Part model, mm, in its own coordinate system. Face numbers are marked on the shaded views. A direction names the side the tool comes from. Round coordinates to 2 decimals unless told otherwise and drop trailing zeros. Loops run counter-clockwise (first coordinate to the right, second up) from the corner with the lowest first, then second, coordinate; pieces in that order, holes last. Notation, with made-up numbers: (45.25, -16) -> (99.25, -16) arc R19 cw to (99.25, 14) -> close; hole circle Ø9 at (56.5, 55). An arc over 180 degrees is marked (long way). Use a Markdown table: item, result. Add a question column.
Item 1: Which spindle directions (+Z, -Z, +X, -X, +Y, -Y) get a long thin tool onto all of the face, cutting with end or side? Do the marked faces 4, 5, 6, 7 and 8. Say none if no direction does.
Item 2: Cut at B-B, the plane y = 17. List the corners of the cut face in (x, z).
Item 3: Probe line 1 (Z direction, x = -94, y = 8); line 2 (X direction, y = 40, z = -35); line 3 (X direction, y = 12, z = -24). List the from-to ranges inside material, lowest first. Write a range as [from, to].
Item 4: Cut at D-D, the plane z = -29.5. List the corners of the cut face in (x, y), plus the area to 3 significant figures.
Item 5: Cut at A-A, the plane x = -80.5. List the corners of the cut face in (y, z).
Item 6: Flat gauge pin, fed straight in: pin 1 (1.5 mm diameter, centred on x = -68.5, z = -37.5, fed in from -Y). Where does the tip first touch, or does it go through?
Item 7: Two-plate mould, pull along X, no slides. Class the marked faces 1, 2 and 3: pulls with the +X half, pulls with the -X half, needs draft (parallel to the pull), parting line crosses it, or undercut.
Item 8: Cut at C-C, the plane z = -48.5. List the corners of the cut face in (x, y).
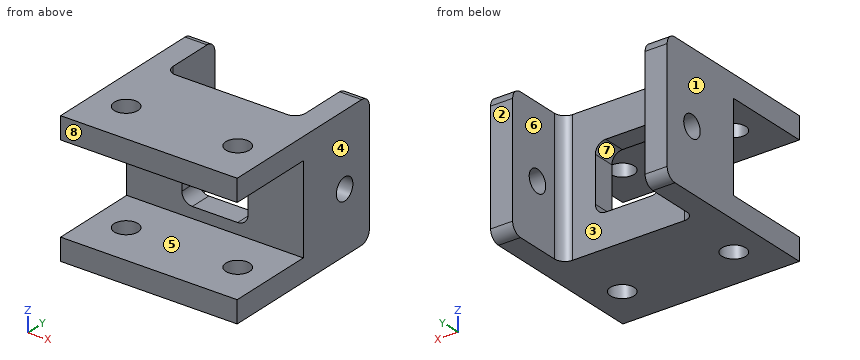
```python
from build123d import *

# Parameters (mm, degrees)
SKETCH1_W               = 50.8
SKETCH1_H               = 38.1
BOSS_EXTRUDE1_DEPTH     = 31.75
SKETCH2_W               = 25.4
SKETCH2_H               = 25.4
CUT_EXTRUDE1_DEPTH      = 85.79053849
SKETCH3_W               = 6.35
SKETCH3_H               = 38.1
BOSS_EXTRUDE2_DEPTH     = 19.05
SKETCH4_W               = 6.35
SKETCH4_H               = 38.1
BOSS_EXTRUDE3_DEPTH     = 19.05
CUT_EXTRUDE2_DEPTH      = 91.317082645
CUT_EXTRUDE2_DEPTH_BACK = 91.317082645
SKETCH5_R               = 3.175
FILLET1_R               = 3
SKETCH6_R               = 3.429
CUT_EXTRUDE3_DEPTH      = 127.788108172
SKETCH7_R               = 3.429
CUT_EXTRUDE4_DEPTH      = 127.788108172
SKETCH8_W               = 19.05
SKETCH8_H               = 19.05
CUT_EXTRUDE5_DEPTH      = 130.041736625
FILLET2_R               = 3
FILLET3_R               = 3


with BuildPart() as part:
    # Sketch1 → Boss-Extrude1 (new body)
    with BuildSketch(Plane(origin=(0, 0, 0), x_dir=(1, 0, 0), z_dir=(0, 1, 0))):
        with Locations((-84.340486484, 40.956107335)):
            Rectangle(SKETCH1_W, SKETCH1_H)
    extrude(amount=BOSS_EXTRUDE1_DEPTH)

    # Sketch2 → Cut-Extrude1 (cut, through all)
    with BuildSketch(Plane(origin=(-58.940486484, 0, 0), x_dir=(0, 0, -1), z_dir=(1, 0, 0))):
        with Locations((40.956107335, 12.7)):
            Rectangle(SKETCH2_W, SKETCH2_H)
    extrude(amount=-CUT_EXTRUDE1_DEPTH, mode=Mode.SUBTRACT)

    # Sketch3 → Boss-Extrude2 (add)
    with BuildSketch(Plane(origin=(0, 31.75, 0), x_dir=(1, 0, 0), z_dir=(0, 1, 0))):
        with Locations((-106.565486484, 40.956107335)):
            Rectangle(SKETCH3_W, SKETCH3_H)
    extrude(amount=BOSS_EXTRUDE2_DEPTH)

    # Sketch4 → Boss-Extrude3 (add)
    with BuildSketch(Plane(origin=(0, 31.75, 0), x_dir=(1, 0, 0), z_dir=(0, 1, 0))):
        with Locations((-62.115486484, 40.956107335)):
            Rectangle(SKETCH4_W, SKETCH4_H)
    extrude(amount=BOSS_EXTRUDE3_DEPTH)

    # Sketch5 → Cut-Extrude2 (cut, two sides: drawn at the far end of the back side and taken through both)
    with BuildSketch(Plane(origin=(-103.390486484, 0, 0), x_dir=(0, 0, -1), z_dir=(1, 0, 0)).offset(-CUT_EXTRUDE2_DEPTH_BACK)):
        with Locations((42.465557169, 41.275)):
            Circle(SKETCH5_R)
    extrude(amount=CUT_EXTRUDE2_DEPTH + CUT_EXTRUDE2_DEPTH_BACK, mode=Mode.SUBTRACT)

    # Fillet1
    fillet1_edges = [part.edges().sort_by_distance(p)[0] for p in [
        (-106.565486484, 50.8, -60.006107335),
        (-106.565486484, 50.8, -21.906107335),
        (-62.115486484, 50.8, -21.906107335),
        (-62.115486484, 50.8, -60.006107335),
        (-65.290486484, 31.75, -40.956107335),
        (-103.390486484, 31.75, -40.956107335),
    ]]
    fillet(fillet1_edges, radius=FILLET1_R)

    # Sketch6 → Cut-Extrude3 (cut, through all)
    with BuildSketch(Plane(origin=(0, 0, -60.006107335), x_dir=(-1, 0, 0), z_dir=(0, 0, -1))):
        with Locations((68.290486484, 12.7)):
            Circle(SKETCH6_R)
    extrude(amount=-CUT_EXTRUDE3_DEPTH, mode=Mode.SUBTRACT)

    # Sketch7 → Cut-Extrude4 (cut, through all)
    with BuildSketch(Plane(origin=(0, 0, -60.006107335), x_dir=(-1, 0, 0), z_dir=(0, 0, -1))):
        with Locations((100.390486484, 12.7)):
            Circle(SKETCH7_R)
    extrude(amount=-CUT_EXTRUDE4_DEPTH, mode=Mode.SUBTRACT)

    # Sketch8 → Cut-Extrude5 (cut, through all)
    with BuildSketch(Plane(origin=(0, 31.75, 0), x_dir=(1, 0, 0), z_dir=(0, 1, 0))):
        with Locations((-84.340486484, 40.956107335)):
            Rectangle(SKETCH8_W, SKETCH8_H)
    extrude(amount=-CUT_EXTRUDE5_DEPTH, mode=Mode.SUBTRACT)

    # Fillet2
    fillet2_edges = [part.edges().sort_by_distance(p)[0] for p in [
        (-93.865486484, 28.575, -31.431107335),
        (-93.865486484, 28.575, -50.481107335),
    ]]
    fillet(fillet2_edges, radius=FILLET2_R)

    # Fillet3
    fillet3_edges = [part.edges().sort_by_distance(p)[0] for p in [
        (-74.815486484, 28.575, -50.481107335),
        (-74.815486484, 28.575, -31.431107335),
    ]]
    fillet(fillet3_edges, radius=FILLET3_R)


solid = part.part
```
A:
| question | item | result |
|---|---|---|
| 1 | face 4 | +Z, -Z, +X, +Y, -Y |
| 1 | face 5 | +X, -X, -Y |
| 1 | face 6 | +Z, -Z, +Y |
| 1 | face 7 | +Y, -Y |
| 1 | face 8 | +Z, -Z, +X, -X, -Y |
| 2 | outline | (-109.74, -60.01) -> (-58.94, -60.01) -> (-58.94, -53.66) -> (-109.74, -53.66) -> close; (-109.74, -28.26) -> (-58.94, -28.26) -> (-58.94, -21.91) -> (-109.74, -21.91) -> close |
| 3 | line 1 | z = [-60.01, -53.66], [-28.26, -21.91] |
| 3 | line 2 | x = [-109.74, -103.39], [-65.29, -58.94] |
| 3 | line 3 | x = [-109.74, -103.75], [-97.03, -71.65], [-64.93, -58.94] |
| 4 | outline | (-109.74, 25.4) -> (-58.94, 25.4) -> (-58.94, 50.8) -> (-65.29, 50.8) -> (-65.29, 34.75) arc R3 cw to (-68.29, 31.75) -> (-100.39, 31.75) arc R3 cw to (-103.39, 34.75) -> (-103.39, 50.8) -> (-109.74, 50.8) -> close |
| 4 | area | 568 mm^2 |
| 5 | outline | (0, -60.01) -> (31.75, -60.01) -> (31.75, -50.48) -> (25.4, -50.48) -> (25.4, -53.66) -> (0, -53.66) -> close; (0, -28.26) -> (25.4, -28.26) -> (25.4, -31.43) -> (31.75, -31.43) -> (31.75, -21.91) -> (0, -21.91) -> close |
| 6 | pin 1 | stops at y = 25.4 |
| 7 | face 1 | pulls with the -X half |
| 7 | face 2 | needs draft |
| 7 | face 3 | undercut |
| 8 | outline | (-109.74, 25.4) -> (-93.69, 25.4) -> (-93.69, 31.75) -> (-100.39, 31.75) arc R3 cw to (-103.39, 34.75) -> (-103.39, 50.8) -> (-109.74, 50.8) -> close; (-74.99, 25.4) -> (-58.94, 25.4) -> (-58.94, 50.8) -> (-65.29, 50.8) -> (-65.29, 34.75) arc R3 cw to (-68.29, 31.75) -> (-74.99, 31.75) -> close |
